Geometry: final body of the model. Coordinates: model frame, mm. A direction names the side the tool comes from. Coordinates: 2 decimals unless noted, no trailing zeros. Loops run counter-clockwise (first coordinate to the right, second up) from the corner with the lowest first, then second, coordinate; pieces in that order, holes last. Notation, with made-up numbers: (56, -37) - (95, -37) arc R20 ccw to (95, -15) - close; hole circle Ø1 at (57.25, 44). An arc over 180 degrees is marked (long way). Write each question's results on one line, items separated by ' | '. Start each with the question number.
from build123d import *

# Parameters (mm, degrees)
F0_W      = 63.9754086733
F0_H      = 32.954
F1_DEPTH  = 7
F2_W      = 51
F2_H      = 32.954
F3_DEPTH  = 19
F4_W      = 40
F4_H      = 10
F5_DEPTH  = 19
F7_DEPTH  = 47.2
F8_R      = 5
F9_W      = 8.3512892127
F9_H      = 18.0645763493
F10_DEPTH = 19
F11_R     = 5


with BuildPart() as f1:
    # F0 (on Front) → F1 (new body)
    with BuildSketch(Plane.XZ):
        Rectangle(F0_W, F0_H)
    extrude(amount=F1_DEPTH)

    # F2 (on face) → F3 (join)
    with BuildSketch(Plane.XZ.offset(7)):
        Rectangle(F2_W, F2_H)
    extrude(amount=F3_DEPTH)

    # F4 (on face) → F5 (cut)
    with BuildSketch(Plane.XZ.offset(26)):
        with Locations((-0.5, -11.477)):
            Rectangle(F4_W, F4_H)
    extrude(amount=-F5_DEPTH, mode=Mode.SUBTRACT)

    # F6 (on face) → F7 (cut)
    with BuildSketch(Plane.XZ.offset(26)):
        with BuildLine():
            Line((15.5, 16.477), (-15.5, 16.477))
            ThreePointArc((-15.5, 16.477), (0, 0), (15.5, 16.477))
        make_face()
    extrude(amount=-F7_DEPTH, mode=Mode.SUBTRACT)

    # F8
    f8_edges = [f1.edges().sort_by_distance(p)[0] for p in [
        (31.987704, -3.5, 16.477),
        (-31.987704, -3.5, 16.477),
    ]]
    fillet(f8_edges, radius=F8_R)

    # F9 (on face) → F10 (cut)
    with BuildSketch(Plane.XZ.offset(26)):
        with Locations((-21.3243553936, 7.4447118254)):
            Rectangle(F9_W, F9_H)
        with Locations((21.3243553936, 7.4447118254)):
            Rectangle(F9_W, F9_H)
    extrude(amount=-F10_DEPTH, mode=Mode.SUBTRACT)

    # F11
    f11_edges = [f1.edges().sort_by_distance(p)[0] for p in [
        (-17.148711, -16.5, -1.587576),
        (17.148711, -16.5, -1.587576),
    ]]
    fillet(f11_edges, radius=F11_R)


solid = f1.part
1) Pin query (flat end, axial travel): pin 1 Ø1.5 at (y, z) = (-17.5, 8) entering from -X; pin 2 Ø4 at (y, z) = (-10.5, 2) entering from -X; pin 3 Ø7.5 at (y, z) = (-14, -7) entering from +X. Return the tip coordinate at first contact, or that it passes through.
2) Section query D-D on z = -8.5. Output: boundary loops of the cut face in (x, y).
3) Section query A-A on y = -4.5. Output: boundary loops of the cut face in (x, z).
4) Access query for faces 1 (the cylindrical face through (18.57, -16.37, -0.08)), 2 (the flat face through (25.5, -16, -9)), 3 (the flat face through (-24, -17, -1.588)). Directions: +Z, -Z, +X, -X, +Y, -Y. A direction counts if a zero-diameter tool reaches every point of the face in a straight line with its end or side. Return the directions, or none.
5) Section query B-B on z = 9. Output: boundary loops of the cut face in (x, y), and give its area (3 significant figures).
6) Section query C-C on x = 0. Output: boundary loops of the cut face in (y, z).
7) Pull-direction query (Z, two-part tool) for faces 4 (the flat face through (0, -4, -16.477)), 5 (the flat face through (20, -6, 16.477)), 6 (the flat face through (-1, -7, -11)); classes: released by +Z, released by -Z, zero draft, split by the parting line, or undercut.
8) Material intervals for line 1 (X direction, y = -19.5, z = -11); line 2 (Y direction, x = 27, z = 4); line 3 (X direction, y = -10.25, z = 12.5), sorted ascending. Write a range as [from, to].
Returned:
1) pin 1: stops at x = -17.15 | pin 2: stops at x = -18.49 | pin 3: stops at x = 25.5
2) outline: (-31.99, -7) - (-25.5, -7) - (-25.5, -26) - (-20.5, -26) - (-20.5, -7) - (19.5, -7) - (19.5, -26) - (25.5, -26) - (25.5, -7) - (31.99, -7) - (31.99, 0) - (-31.99, 0) - close
3) outline: (-31.99, -16.48) - (31.99, -16.48) - (31.99, 11.48) arc R5 ccw to (26.99, 16.48) - (15.5, 16.48) arc R15.53 cw (long way) to (-15.5, 16.48) - (-26.99, 16.48) arc R5 ccw to (-31.99, 11.48) - close
4) face 1: +Z, +X, -Y | face 2: +Z, -Z, +X, -Y | face 3: +Z, -X, -Y
5) outline: (-31.99, -7) - (-17.15, -7) - (-17.15, -26) - (-14.09, -26) - (-14.09, 0) - (-31.99, 0) - close; (14.09, -26) - (17.15, -26) - (17.15, -7) - (31.99, -7) - (31.99, 0) - (14.09, 0) - close | area: 367 mm²
6) outline: (-26, -6.48) - (-7, -6.48) - (-7, -16.48) - (0, -16.48) - (0, 0) - (-26, 0) - close
7) face 4: released by -Z | face 5: released by +Z | face 6: zero draft
8) line 1: x = [-25.5, -20.5], [19.5, 25.5] | line 2: y = [-7, 0] | line 3: x = [-17.15, -15.23], [15.23, 17.15]
